CAD build for the part. Positions are in the model's coordinates, mm. Give positions to 0.01 mm unless a question says otherwise; leave off trailing zeros. Loops run counter-clockwise (first coordinate to the right, second up) from the corner with the lowest first, then second, coordinate; pieces in that order, holes last.
Item 1: Saw through at A-A on x = 62. Give the cut face in (y, z) (3 decimals), plus the area to 3 significant figures.
Item 2: Drop flat-ended pins along their axis: P1, Ø1, axis at y = 38, z = 2, coming from the -X side (3 decimals); P2, Ø1.6, axis at x = 62.5, z = 1.5, coming from the -Y side (3 decimals); P3, Ø1, axis at x = 14, z = 1.5, coming from the +Y side (3 decimals). Give the stop position or say it passes through.
Item 3: Probe probe 1 along Y at (x, z) = (3, 1.45); probe 2 along X at (y, z) = (59, 0.7) (3 decimals). List the from-to ranges inside material, lowest first.
from build123d import *

# Parameters (mm, degrees)
SKETCH1_W            = 76.2
SKETCH1_H            = 76.2
EXTRUDE1_DEPTH       = 3.175
SKETCH3_W            = 3.175
SKETCH3_H            = 12.7
CUT_EXTRUDE1_DEPTH   = 3.175
LPATTERN1_COUNT      = 3
LPATTERN1_PITCH      = 25.4
LPATTERN1_COUNT_DIR2 = 2
LPATTERN1_PITCH_DIR2 = 73.025
SKETCH4_W            = 12.7
SKETCH4_H            = 3.175
CUT_EXTRUDE2_DEPTH   = 3.175
LPATTERN2_COUNT      = 3
LPATTERN2_PITCH      = 25.4
LPATTERN2_COUNT_DIR2 = 2
LPATTERN2_PITCH_DIR2 = 73.025


with BuildPart() as part:
    # Sketch1 → Extrude1 (new body)
    with BuildSketch(Plane.XY):
        with Locations((38.1, 38.1)):
            Rectangle(SKETCH1_W, SKETCH1_H)
    extrude(amount=EXTRUDE1_DEPTH)

    # Sketch3 → Cut-Extrude1 (cut)
    with BuildSketch(Plane.XY.offset(3.175)):
        with Locations((74.6125, 63.5)):
            Rectangle(SKETCH3_W, SKETCH3_H)
    cut_extrude1 = extrude(amount=-CUT_EXTRUDE1_DEPTH, mode=Mode.SUBTRACT)

    # LPattern1: Cut-Extrude1 3 × 2
    with Locations(*[(-j * LPATTERN1_PITCH_DIR2, -i * LPATTERN1_PITCH, 0) for i in range(LPATTERN1_COUNT) for j in range(LPATTERN1_COUNT_DIR2) if (i, j) != (0, 0)]):
        add(cut_extrude1, mode=Mode.SUBTRACT)

    # Sketch4 → Cut-Extrude2 (cut)
    with BuildSketch(Plane.XY.offset(3.175)):
        with Locations((63.5, 74.6125)):
            Rectangle(SKETCH4_W, SKETCH4_H)
    cut_extrude2 = extrude(amount=-CUT_EXTRUDE2_DEPTH, mode=Mode.SUBTRACT)

    # LPattern2: Cut-Extrude2 3 × 2
    with Locations(*[(-i * LPATTERN2_PITCH, -j * LPATTERN2_PITCH_DIR2, 0) for i in range(LPATTERN2_COUNT) for j in range(LPATTERN2_COUNT_DIR2) if (i, j) != (0, 0)]):
        add(cut_extrude2, mode=Mode.SUBTRACT)


solid = part.part
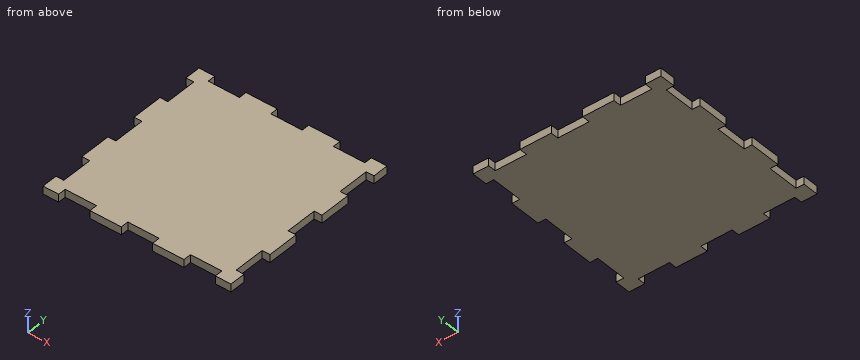
Results below:
1. outline: (3.175, 0) - (73.025, 0) - (73.025, 3.175) - (3.175, 3.175) - close
1. area: 222 mm2
2. P1: stops at x = 3.175
2. P2: stops at y = 3.175
2. P3: stops at y = 73.025
3. probe 1: y = 0 to 6.35, 19.05 to 31.75, 44.45 to 57.15, 69.85 to 76.2
3. probe 2: x = 3.175 to 73.025
